Job drawing, mm, ordinate dimensions from the low corner. One solid piece. A direction names the side the tool comes from. Coordinates: 2 decimals unless noted, no trailing zeros. Write each loop counter-clockwise with the first axis right and the second up, starting at its lowest first coordinate (ties: lowest second). Pieces come first, ordered by that corner, then holes.
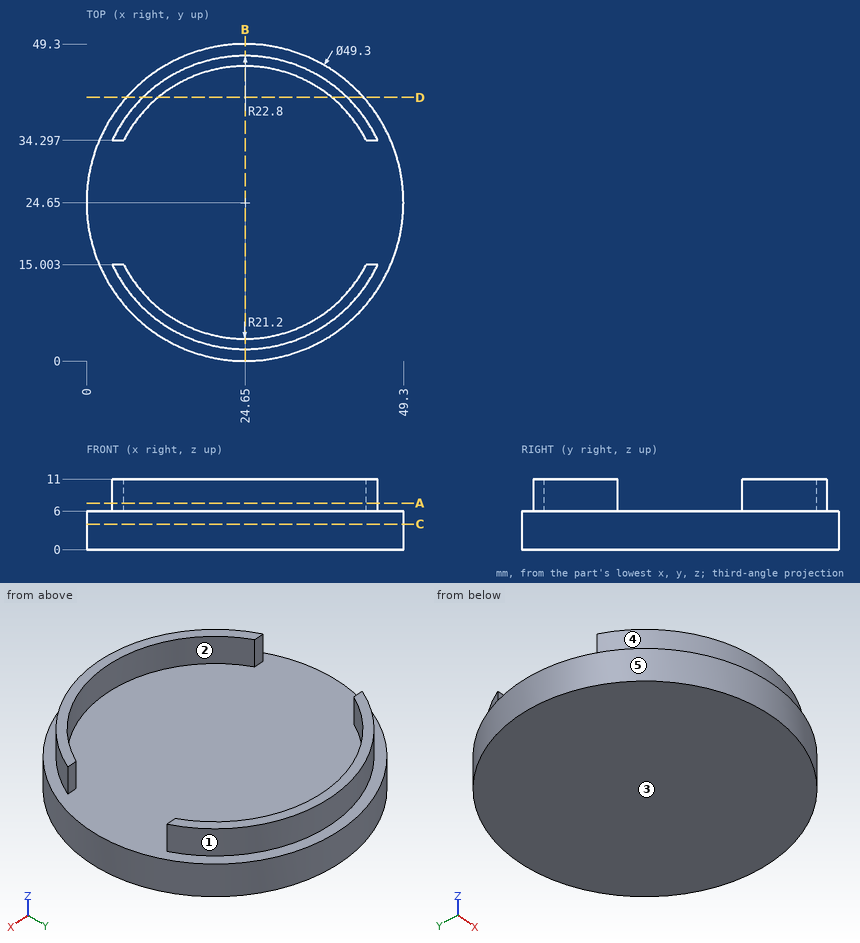
1. Saw through at C-C on z = 4. List the corners of the cut face in (x, y), plus the area to 3 significant figures.
Computed values:
outline: circle Ø49.3 at (24.65, 24.65)
area: 1,910 mm2
2. 3-axis set-ups, long thin cutter, end or side, ignore diameter. For the marked faces 4 and 5: which of +Z, -Z, +X, -X, +Y, -Y reach the whole face in a straight line?
Computed values:
face 4: +Z, -Y
face 5: +Z, -Z
3. Saw through at A-A on z = 7.25. List the corners of the cut face in (x, y), plus the area to 3 significant figures.
Computed values:
outline: (3.99, 15) arc R22.8 ccw to (45.31, 15) - (43.53, 15) arc R21.2 cw to (5.77, 15) - close; (3.99, 34.3) - (5.77, 34.3) arc R21.2 cw to (43.53, 34.3) - (45.31, 34.3) arc R22.8 ccw to start
area: 157 mm2
4. Saw through at D-D on y = 41. List the corners of the cut face in (x, z) (1 decimal), plus the area to 3 significant figures.
Computed values:
outline: (6.2, 0) - (43.1, 0) - (43.1, 6) - (40.5, 6) - (40.5, 11) - (38.1, 11) - (38.1, 6) - (11.2, 6) - (11.2, 11) - (8.8, 11) - (8.8, 6) - (6.2, 6) - close
area: 245 mm2
5. Saw through at B-B on x = 24.65. List the corners of the cut face in (y, z).
Computed values:
outline: (0, 0) - (49.3, 0) - (49.3, 6) - (47.45, 6) - (47.45, 11) - (45.85, 11) - (45.85, 6) - (3.45, 6) - (3.45, 11) - (1.85, 11) - (1.85, 6) - (0, 6) - close
6. Probe line 1 along Z through (x, y) = (40.5, 28); line 2 along Y through (x, z) = (34, 3.75); line 3 along Y through (x, z) = (32, 6.25) (1 decimal). List the from-to ranges inside material, lowest first.
Computed values:
line 1: z = 0 to 6
line 2: y = 1.84 to 47.46
line 3: y = 3.1 to 4.8, 44.5 to 46.2
7. Mould opens along X. For the marked faces 1, 2 and 3 say: +X half, -X half, draft (parallel to the pull), parting line (faces both ways), or undercut.
Computed values:
face 1: parting line
face 2: undercut
face 3: draft
8. Flat gauge pins, fed straight in: pin 1 (0.9 mm diameter, centred on x = 44, z = 8, fed in from +Y); pin 2 (1.5 mm diameter, centred on y = 6, z = 2, fed in from -X); pin 3 (1.4 mm diameter, centred on x = 4.5, z = 7.5, fed in from +Y). Where does each tip first touch, or does it go through?
Computed values:
pin 1: stops at y = 37.4
pin 2: stops at x = 7.7
pin 3: stops at y = 36.55
